from build123d import *

# Parameters (mm, degrees)
SKETCH2_R               = 13.25
BOSS_EXTRUDE1_DEPTH     = 7
SKETCH3_R               = 3.975
CUT_EXTRUDE1_DEPTH      = 5
SKETCH4_W               = 20.55
SKETCH4_H               = 16.05
CUT_EXTRUDE2_DEPTH      = 1
SKETCH5_R               = 1.375
CUT_EXTRUDE3_DEPTH      = 6
FILLET1_R               = 1
CUT_EXTRUDE5_DEPTH      = 1
CUT_EXTRUDE5_DEPTH_BACK = 3
SKETCH6_W               = 20.55
SKETCH6_H               = 8.25
FILLET2_R               = 0.5


with BuildPart() as part:
    # Sketch2 → Boss-Extrude1 (new body)
    with BuildSketch(Plane(origin=(0, 0, 0), x_dir=(1, 0, 0), z_dir=(0, 1, 0))):
        with Locations(Location((0, 0, 0), (0, 0, 270))):
            Circle(SKETCH2_R)
    extrude(amount=BOSS_EXTRUDE1_DEPTH)

    # Sketch3 → Cut-Extrude1 (cut)
    with BuildSketch(Plane(origin=(0, 7, 0), x_dir=(1, 0, 0), z_dir=(0, 1, 0))):
        with Locations(Location((0, 0, 0), (0, 0, 270))):
            Circle(SKETCH3_R)
    extrude(amount=-CUT_EXTRUDE1_DEPTH, mode=Mode.SUBTRACT)

    # Sketch4 → Cut-Extrude2 (cut)
    with BuildSketch(Plane.XZ):
        Rectangle(SKETCH4_W, SKETCH4_H)
    extrude(amount=-CUT_EXTRUDE2_DEPTH, mode=Mode.SUBTRACT)

    # Sketch5 → Cut-Extrude3 (cut)
    with BuildSketch(Plane.XZ.offset(-1)):
        with Locations(Location((-8, -5.725, 0), (0, 0, 270))):
            Circle(SKETCH5_R)
        with Locations(Location((8, -5.725, 0), (0, 0, 270))):
            Circle(SKETCH5_R)
    extrude(amount=-CUT_EXTRUDE3_DEPTH, mode=Mode.SUBTRACT)

    # Fillet1
    fillet1_edges = [part.edges().sort_by_distance(p)[0] for p in [
        (0, 7, -13.25),
    ]]
    fillet(fillet1_edges, radius=FILLET1_R)

    # Sketch6 → Cut-Extrude5 (cut, two sides: drawn at the far end of the back side and taken through both)
    with BuildSketch(Plane.XZ.offset(-1).offset(-CUT_EXTRUDE5_DEPTH_BACK)):
        with Locations((0, 9.125)):
            Rectangle(SKETCH6_W, SKETCH6_H)
    extrude(amount=CUT_EXTRUDE5_DEPTH + CUT_EXTRUDE5_DEPTH_BACK, mode=Mode.SUBTRACT)

    # Fillet2
    fillet2_edges = [part.edges().sort_by_distance(p)[0] for p in [
        (-10.275, 2, 8.36581586),
        (10.275, 2, 8.36581586),
    ]]
    fillet(fillet2_edges, radius=FILLET2_R)


solid = part.part
Could you check a few things on this model? Use its own coordinates, in mm. A direction names the side the tool comes from. Give positions to 0.01 mm unless a question says otherwise; leave off trailing zeros. Order: outer loops, then holes, each group sorted by start corner. A loop starts at its lowest first (then second) coordinate and runs counter-clockwise, first axis right, second up. Notation, with made-up numbers: (77, -26) - (100, -26) arc R11 cw to (100, -16) - close; hole circle Ø2 at (60, 63.5). An arc over 180 degrees is marked (long way). One line per question, with ' | ' between items. Start each with the question number.
Item 1: Thinking about a two-plate mould opening in X: for faces 4 (the cylindrical face through (-6.84, 3.96, -6.46)), 5 (the flat face through (3, 7, -3)), 6 (the cylindrical face through (-2.419, 4.535, -3.154)), 7 (the cylindrical face through (0.583, 2.958, -13.237)), which applies, pulls with the +X half, pulls with the -X half, needs draft (parallel to the pull), parting line crosses it, or undercut?
Item 2: For faces 1 (the flat face through (0.1, 0, -8.3)), 2 (the flat face through (0, 4, 8)), 3 (the flat face through (0, 2, 0)), which set-ups out of +Z, -Z, +X, -X, +Y, -Y let a thin tool reach every point of the face, with its end or its side?
Item 3: I want a section at C-C on y = 2.5. Write out the boundary of the cut face in (x, z) (3 decimals).
Item 4: I'm going to push flat-ended pins straight in: pin 1 Ø2 at (y, z) = (2, -10) entering from +X; pin 2 Ø2 at (x, y) = (3.5, 5) entering from -Z; pin 3 Ø0.5 at (x, y) = (-4, 0.5) entering from +Z (3 decimals); pin 4 Ø2 at (x, z) = (-8, -5.725) entering from -Y. Where does each tip first touch, or does it pass through?
Item 5: I want a section at A-A on x = 0. Write out the boundary of the cut face in (y, z) (3 decimals).
Item 6: I want a section at D-D on y = 4.5. Write out the boundary of the cut face in (x, z) (3 decimals), then the cut area to 3 significant figures.
Item 7: I want a section at B-B on z = 0. Write out the boundary of the cut face in (x, y) (3 decimals), then the cut area to 3 significant figures.
Item 8: I need wall thicknesses on probe 1 along X at (y, z) = (5.6, 0) (3 decimals); probe 2 along X at (y, z) = (3.25, -5.5); probe 3 along X at (y, z) = (4.5, -6.75). Which ranges of each line are inside material? Lowest first, please. Write a range as [from, to].
Verdict:
1) face 4: undercut | face 5: needs draft | face 6: undercut | face 7: parting line crosses it
2) face 1: +Z, -Z, +X, -X, -Y | face 2: +Z, -Y | face 3: +Y
3) outline: (-11.198, 7.084) arc R13.25 ccw (long way) to (11.198, 7.084) arc R0.5 ccw to (10.275, 6.816) - (10.275, 5) - (-10.275, 5) - (-10.275, 6.816) arc R0.5 ccw to start; hole circle Ø2.75 at (-8, -5.725); hole circle Ø7.95 at (0, 0); hole circle Ø2.75 at (8, -5.725)
4) pin 1: x = 9.72 | pin 2: z = -13.01 | pin 3: z = -8.025 | pin 4: through
5) outline: (0, -13.25) - (6, -13.25) arc R1 ccw to (7, -12.25) - (7, -3.975) - (2, -3.975) - (2, 3.975) - (7, 3.975) - (7, 12.25) arc R1 ccw to (6, 13.25) - (4, 13.25) - (4, 5) - (1, 5) - (1, -8.025) - (0, -8.025) - close
6) outline: circle Ø26.5 at (0, 0); hole circle Ø2.75 at (-8, -5.725); hole circle Ø7.95 at (0, 0); hole circle Ø2.75 at (8, -5.725) | area: 490 mm^2
7) outline: (-13.25, 0) - (-10.275, 0) - (-10.275, 1) - (10.275, 1) - (10.275, 0) - (13.25, 0) - (13.25, 6) arc R1 ccw to (12.25, 7) - (3.975, 7) - (3.975, 2) - (-3.975, 2) - (-3.975, 7) - (-12.25, 7) arc R1 ccw to (-13.25, 6) - close | area: 125 mm^2
8) probe 1: [-13.25, -3.975], [3.975, 13.25] | probe 2: [-12.05, -9.36], [-6.64, 6.64], [9.36, 12.05] | probe 3: [-11.4, -8.92], [-7.08, 7.08], [8.92, 11.4]
